The listing builds one solid part. Answer for the finished solid, in the listing's coordinates (mm). A direction names the side the tool comes from. Coordinates: 2 decimals unless noted, no trailing zeros. Write each loop counter-clockwise with the first axis right and the second up, starting at its lowest first coordinate (ties: lowest second). Pieces come first, ordered by that corner, then holes.
(1) The part is cut by section C-C on x = -3.25. Determine the outline of the cut face in (y, z).
(2) Which of the six approach directions +Z, -Z, +X, -X, +Y, -Y give full straight-line access (tool end or side, diameter ignored) to faces 4 (the flat face through (-0.491, 53, 1)), 5 (the flat face through (-10.453, 54, 1))?
(3) Given P1, Ø1.5, axis at y = 55.5, z = 2, coming from the -X side, flat-ended and moving along its own axis, determine where the tip first touches the part or whether it passes through.
(4) For a pull along Y with two mould halves and no side action, classify faces 1 (the flat face through (-6, 46.122, 1)), 2 (the cylindrical face through (-5.743, 55.448, 1.479)), 3 (the flat face through (-6, 54, 3)) as +Y half, -Y half, draft (parallel to the pull), parting line (faces both ways), or undercut.
(5) The part is cut by section A-A on z = 0.75. Determine the outline of the cut face in (x, y).
(6) Straight lines are drawn through the part: line 1 (Y direction, x = -6.5, z = 1.25); line 2 (X direction, y = 53, z = 2.25); line 3 (Y direction, x = -4.75, z = 2.8). For each, find the intervals that lie inside material, in ascending order.
(7) The part is cut by section B-B on x = -8.5. Determine the outline of the cut face in (y, z), plus the area to 3 significant figures.
from build123d import *

# Parameters (mm, degrees)
SKETCH1_R           = 1.25
BOSS_EXTRUDE1_DEPTH = 3


with BuildPart() as part:
    # Sketch1 → Boss-Extrude1 (new body)
    with BuildSketch(Plane.XY):
        with BuildLine():
            Line((-10.453152026, 49.121338482), (-10.49069983, 46.121502107))
            Line((-10.49069983, 46.121502107), (-0.49069983, 46.121502107))
            Line((-0.49069983, 46.121502107), (-0.49069983, 49.121502107))
            Line((-0.49069983, 49.121502107), (-0.49069983, 59.121338482))
            ThreePointArc((-0.49069983, 59.121338482), (-5.471925928, 62.221036999), (-10.453152026, 59.121338482))
            Line((-10.453152026, 59.121338482), (-10.453152026, 49.121338482))
        make_face()
        with Locations((-5.471925928, 56.668764069)):
            Circle(SKETCH1_R, mode=Mode.SUBTRACT)
    extrude(amount=BOSS_EXTRUDE1_DEPTH)


solid = part.part
Model answer:
1. outline: (46.12, 0) - (61.76, 0) - (61.76, 3) - (46.12, 3) - close
2. face 4: +Z, -Z, +X, +Y, -Y
2. face 5: +Z, -Z, -X, +Y
3. P1: stops at x = -10.45
4. face 1: -Y half
4. face 2: undercut
4. face 3: draft
5. outline: (-10.49, 46.12) - (-0.49, 46.12) - (-0.49, 59.12) arc R5.55 ccw to (-10.45, 59.12) - (-10.45, 49.12) - close; hole circle Ø2.5 at (-5.47, 56.67)
6. line 1: y = 46.12 to 55.96, 57.38 to 62.13
6. line 2: x = -10.45 to -0.49
6. line 3: y = 46.12 to 55.65, 57.69 to 62.17
7. outline: (46.12, 0) - (61.32, 0) - (61.32, 3) - (46.12, 3) - close
7. area: 45.6 mm2
